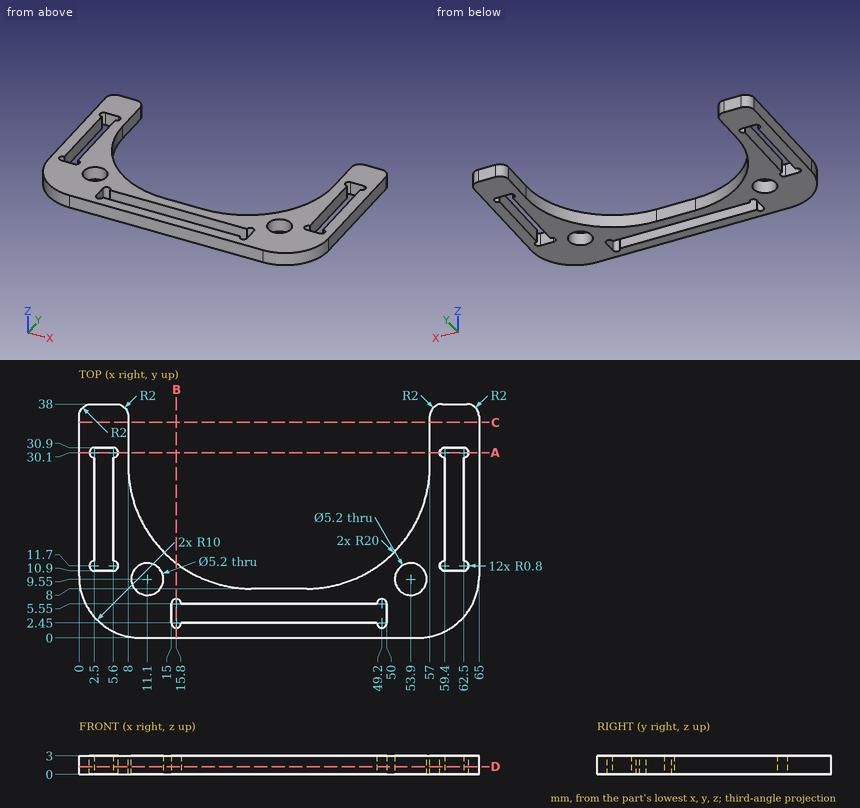
Print and shaded views of the part. All mm, measured from the part's lowest x, y and z. Coordinates: 2 decimals unless noted, no trailing zeros. Write each loop counter-clockwise with the first axis right and the second up, starting at its lowest first coordinate (ties: lowest second). Pieces come first, ordered by that corner, then holes.
(1) Drill centre lines: probe 1 along X at (y, z) = (30, 2.05); probe 2 along X at (y, z) = (28, 1.75); probe 3 along Y at (x, z) = (34, 1.9). Where is each one in solid material? Low to high.
(2) Cut at B-B, the plane x = 15.8. List the corners of the cut face in (y, z), and give its area (3 significant figures).
(3) Cut at A-A, the plane y = 30.1. List the corners of the cut face in (x, z), and give its area (3 significant figures).
(4) Flat gauge pins, fed straight in: pin 1 (6 mm diameter, centred on x = 53.9, y = 9.55, fed in from +Z); pin 2 (1.5 mm diameter, centred on x = 32.5, z = 1.5, fed in from +Y); pin 3 (0.9 mm diameter, centred on x = 61, z = 2, fed in from -Y); pin 4 (0.9 mm diameter, centred on y = 3.5, z = 1.5, fed in from -X). Where does each tip first touch, or does it go through?
(5) Cut at C-C, the plane y = 35. List the corners of the cut face in (x, z).
(6) Cut at D-D, the plane z = 1.25. Count the separate pieces of the cut face and the enclosed holes in it, and give its area (3 significant figures).
Geometry says:
1. probe 1: x = 0 to 1.71, 6.39 to 8, 57 to 58.61, 63.29 to 65
1. probe 2: x = 0 to 2.5, 5.6 to 8, 57 to 59.4, 62.5 to 65
1. probe 3: y = 0 to 2.45, 5.55 to 8
2. outline: (0, 0) - (1.65, 0) - (1.65, 3) - (0, 3) - close; (6.35, 0) - (12.15, 0) - (12.15, 3) - (6.35, 3) - close
2. area: 22.4 mm2
3. outline: (0, 0) - (1.7, 0) - (1.7, 3) - (0, 3) - close; (6.4, 0) - (8, 0) - (8, 3) - (6.4, 3) - close; (57, 0) - (58.6, 0) - (58.6, 3) - (57, 3) - close; (63.3, 0) - (65, 0) - (65, 3) - (63.3, 3) - close
3. area: 19.8 mm2
4. pin 1: stops at z = 3
4. pin 2: stops at y = 8
4. pin 3: stops at y = 1.68
4. pin 4: stops at x = 2.04
5. outline: (0, 0) - (8, 0) - (8, 3) - (0, 3) - close; (57, 0) - (65, 0) - (65, 3) - (57, 3) - close
6. separate pieces: 1
6. enclosed holes: 5
6. area: 838 mm2
